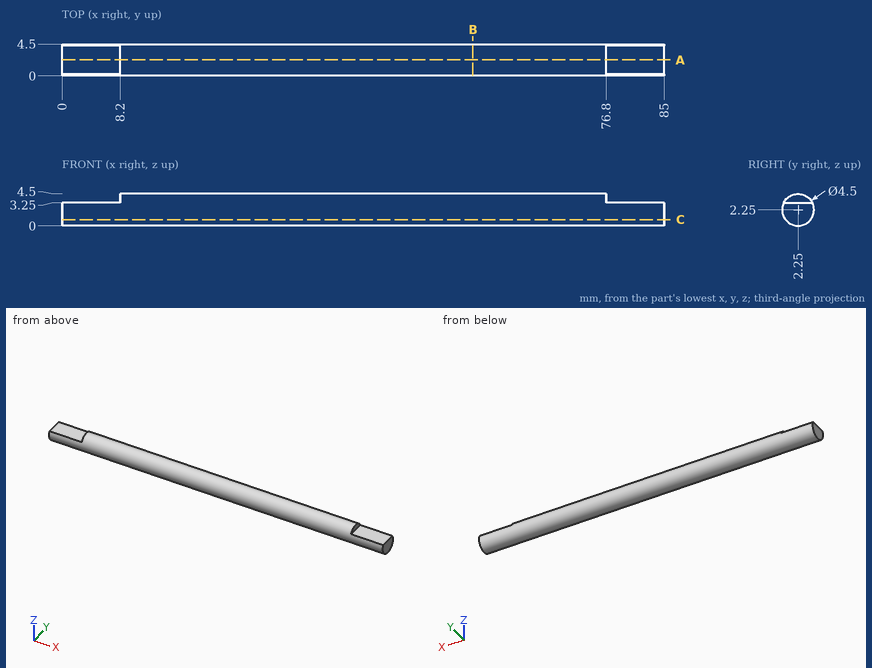
Geometry: see drawing. Coordinates: mm, zero at the bounding-box minimum. Round coordinates to 2 decimals unless told otherwise and drop trailing zeros. Write each loop counter-clockwise with the first axis right and the second up, starting at its lowest first coordinate (ties: lowest second). Pieces come first, ordered by that corner, then holes.
1) Cut plane B-B (x = 58). Return the cut outline in (y, z).
2) Cut plane A-A (y = 2.25). Return the cut outline in (x, z), then the cut area to 3 significant figures.
3) Cut plane C-C (z = 0.85). Return the cut outline in (x, y), then the cut area to 3 significant figures.
4) Ray query, L1, parallel to X at y = 1.9, z = 3.75; L2, parallel to Y at x = 15, z = 2.5; L3, parallel to Z at x = 40, y = 2.1 (3 decimals). Return the intervals inside material, ascending.
5) Contact query for flat-ended pins moving along their axis: P1, Ø1, axis at x = 17.5, z = 2.5, coming from the -Y side; P2, Ø0.6, axis at y = 2, z = 4, coming from the -X side. Output: stop coordinate, or through.
Geometry says:
1. outline: circle Ø4.5 at (2.25, 2.25)
2. outline: (0, 0) - (85, 0) - (85, 3.25) - (76.8, 3.25) - (76.8, 4.5) - (8.2, 4.5) - (8.2, 3.25) - (0, 3.25) - close
2. area: 362 mm2
3. outline: (0, 0.49) - (85, 0.49) - (85, 4.01) - (0, 4.01) - close
3. area: 299 mm2
4. L1: x = 8.2 to 76.8
4. L2: y = 0.01 to 4.49
4. L3: z = 0.005 to 4.495
5. P1: stops at y = 0
5. P2: stops at x = 8.2
